Check sheet for the modelled part. Datum: model origin and axes. Units: mm. Face numbers are marked on the shaded views. A direction names the side the tool comes from. Round coordinates to 2 decimals unless told otherwise and drop trailing zeros. Write each loop counter-clockwise with the first axis right and the second up, starting at its lowest first coordinate (ties: lowest second). Pieces come first, ordered by that corner, then holes. Notation, with made-up numbers: (34, 2.25) - (74, 2.25) arc R11 ccw to (74, 6.25) - close; hole circle Ø4 at (-6, -36). An arc over 180 degrees is marked (long way). Answer as a JSON object with one key per item and string values. Group by question number.
Item 1: Set-up check for the marked faces 1 and 2: record each of +Z, -Z, +X, -X, +Y, -Y from which the full face is reachable in a straight line by a thin tool's end or side.
Item 2: Sectioned sample at D-D on z = -22.5. Record the boundary of the cut face in (x, y).
Item 3: Sectioned sample at B-B on y = 22. Record the boundary of the cut face in (x, z), plus the area to 3 significant figures.
Item 4: Release check for a two-part mould opening along Y. For the marked faces 3, 4 and 5 record: pulls with the +Y half, pulls with the -Y half, needs draft (parallel to the pull), parting line crosses it, or undercut.
Item 5: Gauge pin test, flat ends, axial feed: P1, Ø7, axis at x = 18, y = 6, coming from the +Z side; P2, Ø1, axis at x = 11.5, y = -5.5, coming from the +Z side; P3, Ø6, axis at x = 14, y = -13, coming from the -Z side. Record the tip position at first contact, or that the pin passes through.
Item 6: Sectioned sample at C-C on x = 2.5. Record the boundary of the cut face in (y, z).
Item 7: Sectioned sample at A-A on z = 25.5. Record the boundary of the cut face in (x, y).
Item 8: Thickness scan on line 1 (Z direction, x = 4, y = 5); line 2 (Z direction, x = 8.25, y = 11); line 3 (Z direction, x = 12.5, y = -13). Record the ranges inside material, lowest first.
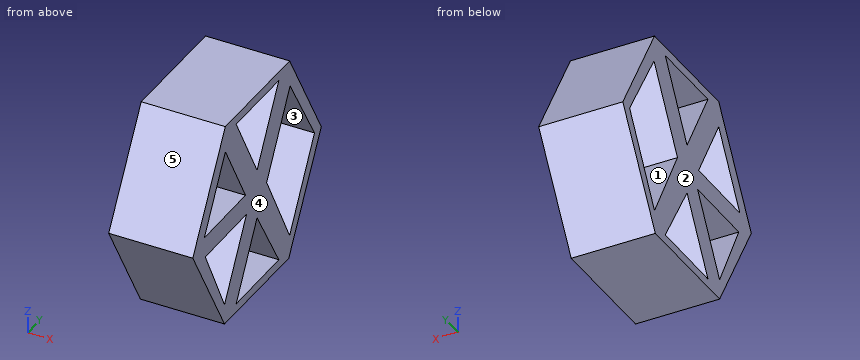
```python
from build123d import *

# Parameters (mm, degrees)
F1_DEPTH = 25.146
F3_DEPTH = 25.147


with BuildPart() as f1:
    # F0 (on Right) → F1 (new body)
    with BuildSketch(Plane.YZ):
        Polygon((-18.196719, -30.976094), (17.727725, -31.246868), (35.924444, -0.270774), (18.196719, 30.976094), (-17.727725, 31.246868), (-35.924444, 0.270774), align=None)
    extrude(amount=F1_DEPTH)

    # F2 (on face) → F3 (cut, through all)
    with BuildSketch(Plane.YZ.offset(25.146)):
        Polygon((12.158216, 28.30131), (-11.682742, 28.481007), (0, 7.056957), align=None)
        Polygon((18.470482, 22.909693), (5.359186, 0), (18.196719, -24.320445), (32.115393, 0), align=None)
        Polygon((12.158216, -28.440368), (0, -8.026823), (-11.682742, -28.440368), align=None)
        Polygon((-5.873994, -3.44487), (-28.931567, -3.44487), (-18.196719, -24.876591), align=None)
        Polygon((-6.465211, 2.910744), (-17.69839, 23.307832), (-29.490458, 2.910744), align=None)
    extrude(amount=-F3_DEPTH, mode=Mode.SUBTRACT)


solid = f1.part
```
Completed:
{
 "1": {"face 1": "+X, -X", "face 2": "+Z, -Z, -X, +Y, -Y"},
 "2": {"outline": "(0, -23.01) - (25.15, -23.01) - (25.15, -19.39) - (0, -19.39) - close; (0, -16.83) - (25.15, -16.83) - (25.15, -8.28) - (0, -8.28) - close; (0, 8.62) - (25.15, 8.62) - (25.15, 17.24) - (0, 17.24) - close; (0, 19.24) - (25.15, 19.24) - (25.15, 22.87) - (0, 22.87) - close"},
 "3": {"outline": "(0, -23.97) - (25.15, -23.97) - (25.15, -17.67) - (0, -17.67) - close; (0, 16.98) - (25.15, 16.98) - (25.15, 24.27) - (0, 24.27) - close", "area": "342 mm²"},
 "4": {"face 3": "undercut", "face 4": "needs draft", "face 5": "pulls with the -Y half"},
 "5": {"P1": "z = 31.09", "P2": "z = 31.16", "P3": "z = -31.04"},
 "6": {"outline": "(-35.92, 0.27) - (-18.2, -30.98) - (17.73, -31.25) - (35.92, -0.27) - (18.2, 30.98) - (-17.73, 31.25) - close; hole (-29.49, 2.91) - (-6.47, 2.91) - (-17.7, 23.31) - close; hole (-28.93, -3.44) - (-18.2, -24.88) - (-5.87, -3.44) - close; hole (-11.68, -28.44) - (12.16, -28.44) - (0, -8.03) - close; hole (-11.68, 28.48) - (0, 7.06) - (12.16, 28.3) - close; hole (5.36, 0) - (18.2, -24.32) - (32.12, 0) - (18.47, 22.91) - close"},
 "7": {"outline": "(0, -21.1) - (25.15, -21.1) - (25.15, -10.06) - (0, -10.06) - close; (0, 10.56) - (25.15, 10.56) - (25.15, 21.3) - (0, 21.3) - close"},
 "8": {"line 1": "-31.15 to -28.44, -16.42 to 15.79, 28.36 to 31.08", "line 2": "-31.2 to -28.44, -26.5 to -10.69, 9.86 to 26.28, 28.31 to 31.03", "line 3": "-31.02 to -15.84, -3.44 to 2.91, 14.78 to 31.21"}
}
